For this review, take the finished solid that the model builds, in its own axes (mm). Round coordinates to 2 decimals unless told otherwise and drop trailing zeros. Order: outer loops, then holes, each group sorted by start corner. A loop starts at its lowest first (then second) coordinate and runs counter-clockwise, first axis right, second up. Notation, with made-up numbers: (-2.75, 56.25) - (17.25, 56.25) arc R26 ccw to (17.25, 83.25) - close; hole circle Ø3 at (49.5, 29). An arc over 180 degrees is marked (long way). One line per question, with ' | ' between items.
```python
from build123d import *

# Parameters (mm, degrees)
SKETCH1_W           = 228.6
SKETCH1_H           = 76.2
BOSS_EXTRUDE1_DEPTH = 3.175
SKETCH3_R           = 2.667
CUT_EXTRUDE2_DEPTH  = 3.175


with BuildPart() as part:
    # Sketch1 → Boss-Extrude1 (new body)
    with BuildSketch(Plane.XY):
        Rectangle(SKETCH1_W, SKETCH1_H)
    extrude(amount=BOSS_EXTRUDE1_DEPTH)

    # Sketch3 → Cut-Extrude2 (cut)
    with BuildSketch(Plane.XY.offset(3.175)):
        with Locations((-101.6, 25.4)):
            Circle(SKETCH3_R)
        with Locations(Location((-101.6, -25.4, 0), (0, 0, 180))):
            Circle(SKETCH3_R)
        with Locations((99.872641584, -25.4)):
            Circle(SKETCH3_R)
        with Locations(Location((99.872641584, 25.4, 0), (0, 0, 180))):
            Circle(SKETCH3_R)
    extrude(amount=-CUT_EXTRUDE2_DEPTH, mode=Mode.SUBTRACT)


solid = part.part
```
(1) We need section A-A on x = -101.6. State the section outline as (y, z) points (3 decimals).
Output values:
outline: (-38.1, 0) - (-28.067, 0) - (-28.067, 3.175) - (-38.1, 3.175) - close; (-22.733, 0) - (22.733, 0) - (22.733, 3.175) - (-22.733, 3.175) - close; (28.067, 0) - (38.1, 0) - (38.1, 3.175) - (28.067, 3.175) - close
(2) Mouldability with a two-part tool opening along Y and no side actions: class faces 1 (the cylindrical face through (-103.72, 23.78, 1.61)), 2 (the flat face through (-2, 1, 0)) as released by +Y, released by -Y, zero draft, split by the parting line, or undercut.
Output values:
face 1: undercut | face 2: zero draft
(3) For probe 1 along X at (y, z) = (25, 1.85); probe 2 along Y at (x, z) = (-101.6, 2.55); probe 3 along X at (y, z) = (-27.5, 1.15), list the stretches that pass through material, from the lowest coordinate up. Write a range as [from, to].
Output values:
probe 1: [-114.3, -104.24], [-98.96, 97.24], [102.51, 114.3] | probe 2: [-38.1, -28.07], [-22.73, 22.73], [28.07, 38.1] | probe 3: [-114.3, -103.24], [-99.96, 98.23], [101.52, 114.3]
(4) We need section B-B on y = 25.4. State the section outline as (x, z) points (3 decimals), plus the area to 3 significant figures.
Output values:
outline: (-114.3, 0) - (-104.267, 0) - (-104.267, 3.175) - (-114.3, 3.175) - close; (-98.933, 0) - (97.206, 0) - (97.206, 3.175) - (-98.933, 3.175) - close; (102.54, 0) - (114.3, 0) - (114.3, 3.175) - (102.54, 3.175) - close | area: 692 mm^2
